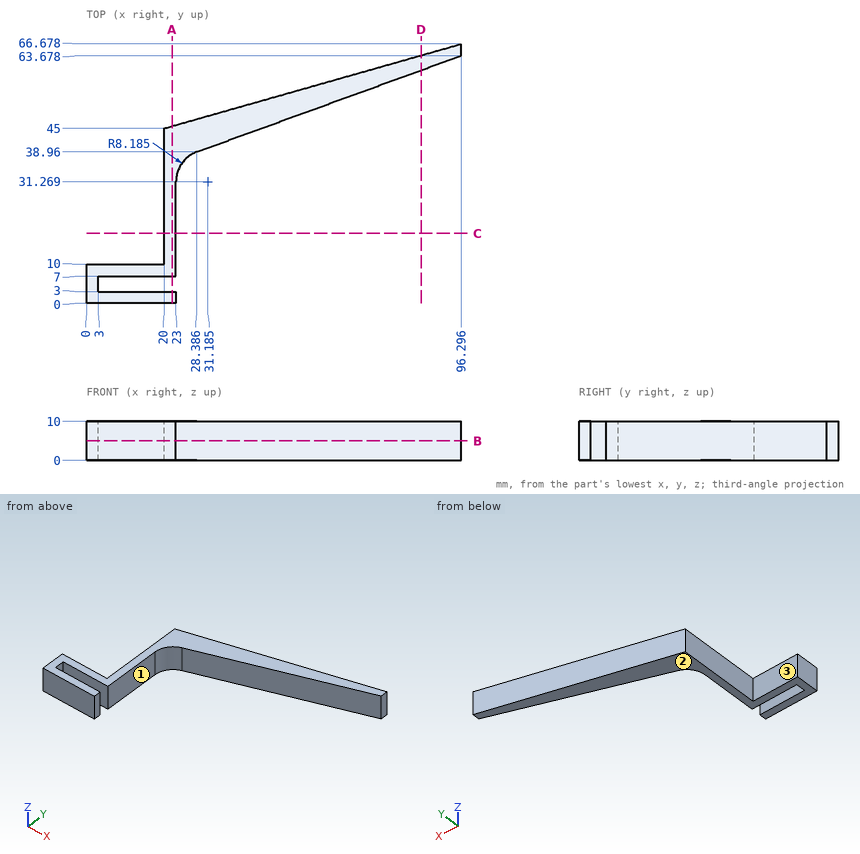
Drawing for the job (mm, zero at the part's lowest x, y, z). A direction names the side the tool comes from. Give positions to 0.01 mm unless a question says otherwise; leave off trailing zeros. Loops run counter-clockwise (first coordinate to the right, second up) from the corner with the lowest first, then second, coordinate; pieces in that order, holes last.
1) Band-saw the part on A-A on x = 22. List the corners of the cut face in (y, z), then the cut area to 3 significant figures.
Values follow:
outline: (0, 0) - (3, 0) - (3, 10) - (0, 10) - close; (7, 0) - (45.57, 0) - (45.57, 10) - (7, 10) - close
area: 416 mm2
2) Band-saw the part on D-D on x = 86. List the corners of the cut face in (y, z).
Values follow:
outline: (59.93, 0) - (63.75, 0) - (63.75, 10) - (59.93, 10) - close
3) Probe line 1 along Y through (x, z) = (4.5, 3.5); line 2 along X through (y, z) = (22.5, 1); line 3 along X through (y, z) = (8, 0.75). List the from-to ranges inside material, lowest first.
Values follow:
line 1: y = 0 to 3, 7 to 10
line 2: x = 20 to 23
line 3: x = 0 to 23
4) 3-axis set-ups, long thin cutter, end or side, ignore diameter. For the marked faces 1, 2 and 3: which of +Z, -Z, +X, -X, +Y, -Y reach the whole face in a straight line?
Values follow:
face 1: +Z, -Z, +X, -Y
face 2: -Z, +X, -X, +Y, -Y
face 3: +Z, -Z, -X, +Y
5) Band-saw the part on C-C on y = 18. List the corners of the cut face in (x, z).
Values follow:
outline: (20, 0) - (23, 0) - (23, 10) - (20, 10) - close
6) Drop flat-ended pins along their axis: P1, Ø10, axis at x = 17.5, y = 50, coming from the -Z side; P2, Ø5, axis at y = 30.5, z = 4.5, coming from the +X side (1 decimal); P3, Ø1.5, axis at y = 1.5, z = 4, coming from the +X side; P4, Ø5, axis at x = 13.5, z = 6.5, coming from the +Y side. Give the stop position or say it passes through.
Values follow:
P1: passes through
P2: stops at x = 23.2
P3: stops at x = 23
P4: stops at y = 10
7) Band-saw the part on B-B on z = 5. List the corners of the cut face in (x, y) (1 decimal).
Values follow:
outline: (0, 0) - (23, 0) - (23, 3) - (3, 3) - (3, 7) - (23, 7) - (23, 31.3) arc R8.2 cw to (28.4, 39) - (96.3, 63.7) - (96.3, 66.7) - (20, 45) - (20, 10) - (0, 10) - close
